Could you check a few things on this model? Use its own coordinates, in mm. A direction names the side the tool comes from. Coordinates: 2 decimals unless noted, no trailing zeros. Loops run counter-clockwise (first coordinate to the right, second up) from the corner with the lowest first, then second, coordinate; pieces in that order, holes last. Notation, with made-up numbers: (-38.75, -29.75) - (18.25, -29.75) arc R29 cw to (18.25, 7.25) - close; hole circle Ø5 at (65, -39). An arc over 180 degrees is marked (long way). One line per item, written item: value. Start each with the question number.
(1) If we section it at B-B on x = 0: Write out the boundary of the cut face in (y, z), then the cut area to 3 significant figures.
(2) If we section it at C-C on z = 11.5: Write out the boundary of the cut face in (x, y).
(3) I'm going to push flat-ended pins straight in: P1, Ø1.5, axis at y = 35, z = -19.5, coming from the -X side; P2, Ø1.5, axis at x = 17.5, y = 24.5, coming from the +Z side; P3, Ø1.3, axis at x = 23.5, y = 53, coming from the +Z side. Where does each tip first touch, or does it pass through?
(4) If we mould it in two halves opening along Z, with no side actions, what happens to faces 4 (the face through (0, 0, 0)), 5 (the face through (23.846, 39.44, -7.509)), 6 (the face through (-0.46, 47.045, 22.495))? For each: pulls with the +Z half, pulls with the -Z half, needs draft (parallel to the pull), parting line crosses it, or undercut.
(5) If we section it at D-D on z = 3.5: Write out the boundary of the cut face in (x, y), then the cut area to 4 significant figures.
(6) On a 3-axis mill with a long thin cutter (end or side, diameter ignored), from which of +Z, -Z, +X, -X, +Y, -Y can I reach the whole of each face in a straight line? I mean faces 1 (the face through (0, 5, 0)), 2 (the face through (24, 48, -2.5)), 3 (the face through (0, 80, 23)). Say none if no direction works.
(7) If I drill on line 1 along X through (y, z) = (7.5, 0); line 2 along Y through (x, z) = (19, 7.5); line 3 along Z through (x, y) = (8.5, 30), over which ranges is the centre line in solid material (lowest first)? Write a range as from..to.
```python
from build123d import *

# Parameters (mm, degrees)
SKETCH1_R           = 25
SKETCH1_R_2         = 22.5
BOSS_EXTRUDE1_DEPTH = 80
SKETCH2_R           = 25
BOSS_EXTRUDE2_DEPTH = 15
SKETCH3_W           = 50
SKETCH3_H           = 5
CUT_EXTRUDE1_DEPTH  = 65
SKETCH4_R           = 5
CUT_EXTRUDE2_DEPTH  = 10


with BuildPart() as part:
    # Sketch1 → Boss-Extrude1 (new body)
    with BuildSketch(Plane(origin=(0, 0, 0), x_dir=(1, 0, 0), z_dir=(0, 1, 0))):
        Circle(SKETCH1_R)
        Circle(SKETCH1_R_2, mode=Mode.SUBTRACT)
    extrude(amount=BOSS_EXTRUDE1_DEPTH)

    # Sketch2 → Boss-Extrude2 (add)
    with BuildSketch(Plane.XZ):
        Circle(SKETCH2_R)
    extrude(amount=-BOSS_EXTRUDE2_DEPTH)

    # Sketch3 → Cut-Extrude1 (cut)
    with BuildSketch(Plane(origin=(0, 80, 0), x_dir=(1, 0, 0), z_dir=(0, 1, 0))):
        Rectangle(SKETCH3_W, SKETCH3_H)
    extrude(amount=-CUT_EXTRUDE1_DEPTH, mode=Mode.SUBTRACT)

    # Sketch4 → Cut-Extrude2 (cut)
    with BuildSketch(Plane(origin=(0, 15, 0), x_dir=(1, 0, 0), z_dir=(0, 1, 0))):
        Circle(SKETCH4_R)
    extrude(amount=-CUT_EXTRUDE2_DEPTH, mode=Mode.SUBTRACT)


solid = part.part
```
Values:
1. outline: (0, -25) - (80, -25) - (80, -22.5) - (15, -22.5) - (15, -5) - (5, -5) - (5, 5) - (15, 5) - (15, 22.5) - (80, 22.5) - (80, 25) - (0, 25) - close
1. area: 975 mm2
2. outline: (-22.2, 0) - (22.2, 0) - (22.2, 80) - (19.34, 80) - (19.34, 15) - (-19.34, 15) - (-19.34, 80) - (-22.2, 80) - close
3. P1: stops at x = -16.54
3. P2: stops at z = 18.56
3. P3: stops at z = 10.14
4. face 4: needs draft
4. face 5: parting line crosses it
4. face 6: undercut
5. outline: (-24.75, 0) - (24.75, 0) - (24.75, 80) - (22.23, 80) - (22.23, 15) - (3.57, 15) - (3.57, 5) - (-3.57, 5) - (-3.57, 15) - (-22.23, 15) - (-22.23, 80) - (-24.75, 80) - close
5. area: 1,000 mm2
6. face 1: +Y
6. face 2: +X, -X, +Y
6. face 3: +Z, -Z, +X, -X, +Y
7. line 1: x = -25..-5, 5..25
7. line 2: y = 0..15
7. line 3: z = -23.51..-20.83, 20.83..23.51
